Input: part model. Units: mm. Frame: model coordinates. Coordinates: 2 decimals unless noted, no trailing zeros. Write each loop counter-clockwise with the first axis right and the second up, starting at its lowest first coordinate (ties: lowest second). Pieces come first, ordered by that corner, then holes. Notation, with made-up numbers: (23.25, -22.75) - (29.25, -22.75) arc R24 cw to (29.25, 0.25) - close; hole circle Ø6 at (5.5, 14). An arc over 180 degrees is marked (long way). Use a Markdown table: item, result. Add a question column.
Q1. Section query B-B (x = 0). Return the cut outline in (y, z), then the cut area to 3 significant figures.
Q2. Section query A-A (y = 0). Return the cut outline in (x, z), then the cut area to 3 significant figures.
Q3. Material intervals for probe 1 along Y at (x, z) = (0, 1.5); probe 2 along X at (y, z) = (0, 2.6); probe 3 along Y at (x, z) = (-1.5, 2.25), sorted ascending. Write a range as from..to.
Q4. Mould query, pull axis X, two halves, no side actions, for faces 1 (the face through (14.859, 0.07, 4.797)), 2 (the face through (-6.02, 0.07, 1.25)), 3 (the face through (8, 0, 3)), 4 (the face through (-16, 0, 1)). Classes: released by +X, released by -X, zero draft, split by the parting line, or undercut.
Q5. Section query D-D (y = 3.75). Return the cut outline in (x, z).
Q6. Section query C-C (z = 2.5). Return the cut outline in (x, y), then the cut area to 3 significant figures.
from build123d import *

# Parameters (mm, degrees)
SKETCH1_W               = 32
SKETCH1_H               = 10
BOSS_EXTRUDE1_DEPTH     = 6
FILLET1_R               = 4
SKETCH3_R               = 1.25
SKETCH3_R_2             = 3
CUT_EXTRUDE1_DEPTH      = 6
CUT_EXTRUDE1_DEPTH_BACK = 6
FILLET2_R               = 0.5


with BuildPart() as part:
    # Sketch1 → Boss-Extrude1 (new body)
    with BuildSketch(Plane.XY):
        Rectangle(SKETCH1_W, SKETCH1_H)
    extrude(amount=BOSS_EXTRUDE1_DEPTH)

    # Fillet1
    fillet1_edges = [part.edges().sort_by_distance(p)[0] for p in [
        (-16, 0, 6),
        (16, 0, 6),
    ]]
    fillet(fillet1_edges, radius=FILLET1_R)

    # Sketch2 → Cut-Revolve1 (revolve, cut)
    with BuildSketch(Plane(origin=(0, 0, 0), x_dir=(1, 0, 0), z_dir=(0, 1, 0))):
        Polygon((3.15, -6), (0, -6), (0, 0), (1.7, 0), (1.7, -4.55), align=None)
    revolve(axis=Axis((0, 0, 12.35), (0, 0, -1)), mode=Mode.SUBTRACT)

    # Sketch3 → Cut-Extrude1 (cut, two sides)
    with BuildSketch(Plane(origin=(0, 0, 0), x_dir=(1, 0, 0), z_dir=(0, 1, 0))) as cut_extrude1_sk:
        with Locations((-11, 0)):
            Circle(SKETCH3_R)
        with Locations((-6, 0)):
            Circle(SKETCH3_R)
        with Locations((8, 0)):
            Circle(SKETCH3_R_2)
    extrude(amount=CUT_EXTRUDE1_DEPTH, mode=Mode.SUBTRACT)
    extrude(cut_extrude1_sk.sketch, amount=-CUT_EXTRUDE1_DEPTH_BACK, mode=Mode.SUBTRACT)

    # Fillet2
    fillet2_edges = [part.edges().sort_by_distance(p)[0] for p in [
        (11, 0, 0),
        (5, 0, 0),
        (-4.75, 0, 0),
        (-7.25, 0, 0),
        (-9.75, 0, 0),
        (-12.25, 0, 0),
    ]]
    fillet(fillet2_edges, radius=FILLET2_R)


solid = part.part
Values follow:
| question | item | result |
|---|---|---|
| 1 | outline | (-5, 0) - (-1.7, 0) - (-1.7, 4.55) - (-3.15, 6) - (-5, 6) - close; (1.7, 0) - (5, 0) - (5, 6) - (3.15, 6) - (1.7, 4.55) - close |
| 1 | area | 37.5 mm2 |
| 2 | outline | (-16, 0) - (-12.68, 0) arc R0.5 ccw to (-12.2, 0.36) arc R1.25 cw to (-9.8, 0.36) arc R0.5 ccw to (-9.32, 0) - (-7.68, 0) arc R0.5 ccw to (-7.2, 0.36) arc R1.25 cw to (-4.8, 0.36) arc R0.5 ccw to (-4.32, 0) - (-1.7, 0) - (-1.7, 4.55) - (-3.15, 6) - (-12, 6) arc R4 ccw to (-16, 2) - close; (1.7, 0) - (4.54, 0) arc R0.5 ccw to (5.03, 0.43) arc R3 cw to (10.97, 0.43) arc R0.5 ccw to (11.46, 0) - (16, 0) - (16, 2) arc R4 ccw to (12, 6) - (3.15, 6) - (1.7, 4.55) - close |
| 2 | area | 143 mm2 |
| 3 | probe 1 | -5..-1.7, 1.7..5 |
| 3 | probe 2 | -15.95..-1.7, 1.7..6.5, 9.5..15.95 |
| 3 | probe 3 | -5..-0.8, 0.8..5 |
| 4 | face 1 | released by +X |
| 4 | face 2 | undercut |
| 4 | face 3 | undercut |
| 4 | face 4 | released by -X |
| 5 | outline | (-16, 0) - (-12.68, 0) arc R0.5 ccw to (-12.2, 0.36) arc R1.25 cw to (-9.8, 0.36) arc R0.5 ccw to (-9.32, 0) - (-7.68, 0) arc R0.5 ccw to (-7.2, 0.36) arc R1.25 cw to (-4.8, 0.36) arc R0.5 ccw to (-4.32, 0) - (4.54, 0) arc R0.5 ccw to (5.03, 0.43) arc R3 cw to (10.97, 0.43) arc R0.5 ccw to (11.46, 0) - (16, 0) - (16, 2) arc R4 ccw to (12, 6) - (-12, 6) arc R4 ccw to (-16, 2) - close |
| 6 | outline | (-15.97, -5) - (6.34, -5) - (6.34, 5) - (-15.97, 5) - close; (9.66, -5) - (15.97, -5) - (15.97, 5) - (9.66, 5) - close; hole circle Ø3.4 at (0, 0) |
| 6 | area | 277 mm2 |
